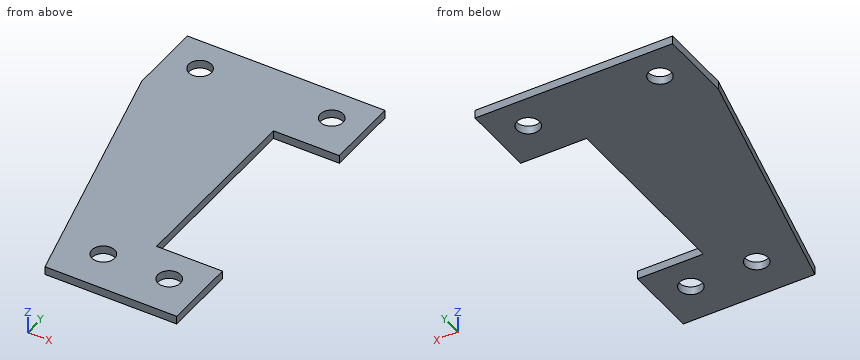
Autodesk Inventor part; units mm, degrees
ref_plane "YZ Plane" through (0, 0, 0) normal (1, 0, 0) x (0, 1, 0)
ref_plane "XZ Plane" through (0, 0, 0) normal (0, 1, 0) x (-1, 0, 0)
ref_plane "XY Plane" through (0, 0, 0) normal (0, 0, 1) x (1, 0, 0)
sketch "Sketch1" plane through (0, 0, 0) normal (0, 0, 1) x (1, 0, 0)
  line L0 (-15.6363, 35.4419) -> (22.4637, 35.4419)
  line L1 (22.4637, 35.4419) -> (22.4637, 21.1544)
  line L2 (22.4637, -15.3581) -> (22.4637, -29.6456)
  line L3 (-2.9363, -29.6456) -> (-15.6363, 21.1544)
  line L4 (22.4637, 21.1544) -> (9.7637, 21.1544)
  line L5 (9.7637, 21.1544) -> (9.7637, -15.3581)
  line L6 (-15.6363, 35.4419) -> (-15.6363, 21.1544)
  line L7 (22.4637, -15.3581) -> (9.7637, -15.3581)
  line L8 (22.4637, -29.6456) -> (-2.9363, -29.6456)
  circle A0 centre (16.1137, 29.0919) radius 2.1844
  circle A1 centre (-9.2863, 29.0919) radius 2.1844
  circle A2 centre (16.1137, -21.7081) radius 2.1844
  circle A3 centre (3.4137, -21.7081) radius 2.1844
  point P0 (0, 0)
  dimension "d0" = 38.1
  dimension "d1" = 12.7
extrude "Extrusion1" add sketch "Sketch1" along normal blind 1.5875
properties part number "FrontFunnelTop"
Source: CAD feature listing. Evaluate the final solid. Frame: model axes, mm. Give positions to 0.01 mm unless a question says otherwise; leave off trailing zeros. Order: outer loops, then holes, each group sorted by start corner. A loop starts at its lowest first (then second) coordinate and runs counter-clockwise, first axis right, second up.
(1) Section query D-D (x = -6). Return the cut outline in (y, z).
(2) Section query A-A (x = 10.5). Return the cut outline in (y, z), plus the area to 3 significant figures.
(3) Contact query for a flat-ended pin moving along its axis: P1, Ø4, axis at x = -9.29, y = 29.09, coming from the +Z side. Output: stop coordinate, or through.
(4) Section query B-B (z = 0.45). Return the cut outline in (x, y).
(5) Section query C-C (y = 1.5). Return the cut outline in (x, z).
(6) Material intervals for line 1 along X through (y, z) = (-21, 1.1); line 2 along Y through (x, z) = (21, 0.6); line 3 along X through (y, z) = (30, 0.6), sorted ascending.
Outcome:
1. outline: (-17.39, 0) - (35.44, 0) - (35.44, 1.59) - (-17.39, 1.59) - close
2. outline: (-29.65, 0) - (-15.36, 0) - (-15.36, 1.59) - (-29.65, 1.59) - close; (21.15, 0) - (35.44, 0) - (35.44, 1.59) - (21.15, 1.59) - close
2. area: 45.4 mm2
3. P1: passes through
4. outline: (-15.64, 21.15) - (-2.94, -29.65) - (22.46, -29.65) - (22.46, -15.36) - (9.76, -15.36) - (9.76, 21.15) - (22.46, 21.15) - (22.46, 35.44) - (-15.64, 35.44) - close; hole circle Ø4.37 at (-9.29, 29.09); hole circle Ø4.37 at (3.41, -21.71); hole circle Ø4.37 at (16.11, -21.71); hole circle Ø4.37 at (16.11, 29.09)
5. outline: (-10.72, 0) - (9.76, 0) - (9.76, 1.59) - (-10.72, 1.59) - close
6. line 1: x = -5.1 to 1.35, 5.48 to 14.05, 18.18 to 22.46
6. line 2: y = -29.65 to -15.36, 21.15 to 35.44
6. line 3: x = -15.64 to -11.27, -7.3 to 14.13, 18.1 to 22.46
